Answer from the drawing. Dimensions are ordinates in mm from the lowest x, y and z of the part. Coordinates: 2 decimals unless noted, no trailing zeros. Write each loop counter-clockwise with the first axis right and the second up, starting at its lowest first coordinate (ties: lowest second). Pieces come first, ordered by that corner, then holes.
(1) Given pin 1 (1.5 mm diameter, centred on x = 33.5, z = 5.5, fed in from -Y); pin 2 (1.5 mm diameter, centred on x = 22.5, y = 1, fed in from -Z), each flat-ended and moving along its own axis, determine where each tip first touches the part or whether it passes through.
(2) The mould has two halves that part along X. Classify the marked faces 1, 2 and 3: +X half, -X half, draft (parallel to the pull), parting line (faces both ways), or undercut.
(3) Section A-A on x = 59 is taken. Write down the section's boundary in (y, z).
(4) Find the intervals of material crossed by probe 1 along Z at (x, y) = (47.5, 2.05) (1 decimal); probe 2 along Z at (x, y) = (5.5, 1.4) (1 decimal); probe 3 along Y at (x, z) = (73, 3.75), in increasing order.
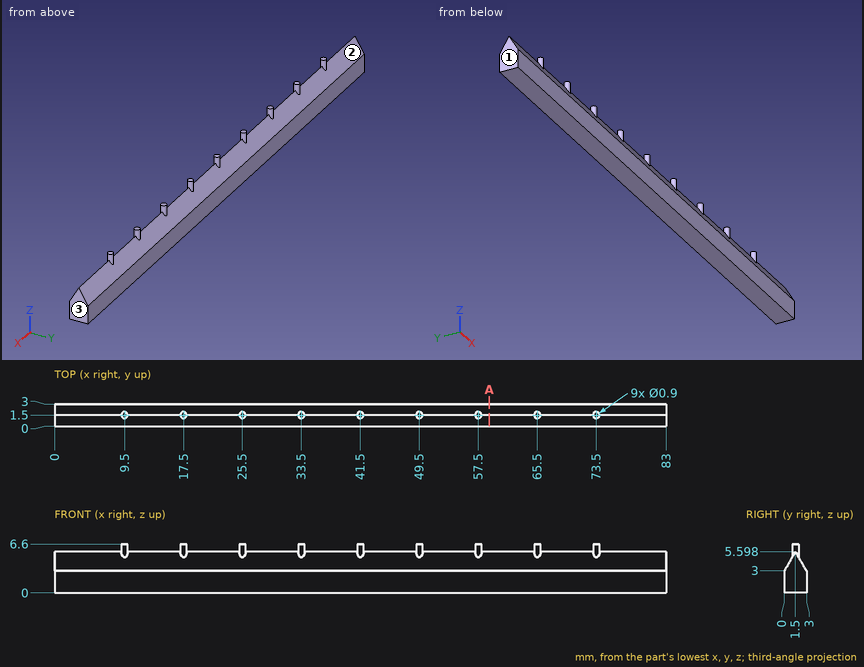
Response:
1. pin 1: stops at y = 1.01
1. pin 2: stops at z = 0
2. face 1: -X half
2. face 2: undercut
2. face 3: +X half
3. outline: (0, 0) - (3, 0) - (3, 3) - (1.5, 5.6) - (0, 3) - close
4. probe 1: z = 0 to 4.6
4. probe 2: z = 0 to 5.4
4. probe 3: y = 0.43 to 2.57
